Geometry check sheet. Reference: the model listing, model coordinates, mm. A direction names the side the tool comes from. Coordinates: 2 decimals unless noted, no trailing zeros. Write each loop counter-clockwise with the first axis right and the second up, starting at its lowest first coordinate (ties: lowest second). Pieces come first, ordered by that corner, then holes. Notation, with made-up numbers: M -7,-18.75 L 19,-18.75 A16 cw 19,8.25 Z; hole C 46.25,-35.75 d7. An arc over 180 degrees is marked long. Put each result on its own line as item: value. Start each with the question number.
1) Set-up check for faces 5 (the flat face through (-31.5, 1.4, 25.7)), 6 (the flat face through (-9.563, 1.401, 22.927)), 7 (the flat face through (-9.563, -1.401, 22.927)): record each of +Z, -Z, +X, -X, +Y, -Y from which the full face is reachable in a straight line by a thin tool's end or side.
2) Scan lines: line 1 along Y through (x, z) = (-2.5, -5.5); line 2 along Y through (x, z) = (-16, 17). Record each from-to range of solid material in increasing order.
3) Gauge pin test, flat ends, axial feed: pin 1 (1 mm diameter, centred on x = -0.5, z = 5.5, fed in from -Y); pin 2 (12 mm diameter, centred on x = -1, z = -2, fed in from -Y); pin 3 (1.5 mm diameter, centred on x = -41.5, y = -1.5, fed in from -Z). Record the tip position at first contact, or that the pin passes through.
4) Mould release check, pull along X, two halves, no side actions. Record for faces 1 (the flat face through (-9.52, -1.98, -1.27)), 2 (the flat face through (-4.314, -1.586, 21.033)), 3 (the flat face through (-10.107, 1.586, 21.141)), 4 (the flat face through (17.372, -1.586, 24.768)): released by +X, released by -X, zero draft, split by the parting line, or undercut.
5) Cross-section at B-B on z = -1. Record the cut outline in (x, y), plus the area to 3 significant figures.
6) Cross-section at A-A on z = 25.5. Count the separate pieces of the cut face and the enclosed holes in it, plus the area to 3 significant figures.
from build123d import *


with BuildPart() as f3:
    # F0 (on Front) → F3 section 0
    with BuildSketch(Plane.XZ, mode=Mode.PRIVATE) as f3_s0:
        with BuildLine():
            Line((-21.9142735004, 32.6593369246), (-64.6117627621, 32.6593369246))
            add(Edge.make_bspline(
                [(-64.6117627621, 32.6593369246), (-63.1112154786, 31.6044133494), (-59.4897111338, 29.4798106269), (-54.8402694545, 24.0083886157), (-54.1776311477, 17.803548493), (-53.0184023082, 15.6934484839)],
                knots=[0, 0, 0, 0, 0.3044179075, 0.6380886555, 1, 1, 1, 1], degree=3))
            add(Edge.make_bspline(
                [(-53.0184023082, 15.6934484839), (-50.397152359, 15.9517944961), (-42.4564652069, 16.5735141568), (-30.3318480055, 11.9726995365), (-22.6326325716, 7.7807102957), (-19.3285813991, 1.5879180834), (-17.1072725207, 0)],
                knots=[0, 0, 0, 0, 0.2494885994, 0.5320392712, 0.7637954486, 1, 1, 1, 1], degree=3))
            Line((-17.1072725207, 0), (-7.2105028667, -11.7347398773))
            Line((-7.2105028667, -11.7347398773), (2.6862667874, 0))
            add(Edge.make_bspline(
                [(38.5973965749, 15.6934484839), (35.9761466257, 15.9517944961), (28.0354594736, 16.5735141568), (15.9108422722, 11.9726995365), (8.2116268383, 7.7807102957), (4.9075756658, 1.5879180834), (2.6862667874, 0)],
                knots=[0, 0, 0, 0, 0.2494885994, 0.5320392712, 0.7637954486, 1, 1, 1, 1], degree=3))
            add(Edge.make_bspline(
                [(50.1907570288, 32.6593369246), (48.6902097453, 31.6044133494), (45.0687054005, 29.4798106269), (40.4192637212, 24.0083886157), (39.7566254144, 17.803548493), (38.5973965749, 15.6934484839)],
                knots=[0, 0, 0, 0, 0.3044179075, 0.6380886555, 1, 1, 1, 1], degree=3))
            Line((50.1907570288, 32.6593369246), (7.4932677671, 32.6593369246))
            add(Edge.make_bspline(
                [(7.4932677671, 32.6593369246), (7.7789275206, 30.681626577), (8.3182882425, 26.9541985329), (4.3276740221, 24.1005648406), (-0.3013873529, 24.1408897918), (-2.9690302908, 24.1763927042)],
                knots=[0, 0, 0, 0, 0.3305961482, 0.6143190537, 1, 1, 1, 1], degree=3))
            Line((-2.9690302908, 24.1763927042), (-2.9690302908, 30.962748453))
            Line((-2.9690302908, 30.962748453), (-4.662130028, 27.2415857762))
            Line((-4.662130028, 27.2415857762), (-7.2105028667, 27.2415857762))
            Line((-7.2105028667, 27.2415857762), (-9.7588757053, 27.2415857762))
            Line((-9.7588757053, 27.2415857762), (-11.4519754425, 30.962748453))
            Line((-11.4519754425, 30.962748453), (-11.4519754425, 24.1763927042))
            add(Edge.make_bspline(
                [(-21.9142735004, 32.6593369246), (-22.199933254, 30.681626577), (-22.7392939758, 26.9541985329), (-18.7486797554, 24.1005648406), (-14.1196183804, 24.1408897918), (-11.4519754425, 24.1763927042)],
                knots=[0, 0, 0, 0, 0.3305961482, 0.6143190537, 1, 1, 1, 1], degree=3))
        make_face()
    loft([f3_s0.sketch, Vertex(-7.2105028667, -5, 7.7760326676)])

    # F0 (on Front) → F6 section 0
    with BuildSketch(Plane.XZ, mode=Mode.PRIVATE) as f6_s0:
        with BuildLine():
            Line((-21.9142735004, 32.6593369246), (-64.6117627621, 32.6593369246))
            add(Edge.make_bspline(
                [(-64.6117627621, 32.6593369246), (-63.1112154786, 31.6044133494), (-59.4897111338, 29.4798106269), (-54.8402694545, 24.0083886157), (-54.1776311477, 17.803548493), (-53.0184023082, 15.6934484839)],
                knots=[0, 0, 0, 0, 0.3044179075, 0.6380886555, 1, 1, 1, 1], degree=3))
            add(Edge.make_bspline(
                [(-53.0184023082, 15.6934484839), (-50.397152359, 15.9517944961), (-42.4564652069, 16.5735141568), (-30.3318480055, 11.9726995365), (-22.6326325716, 7.7807102957), (-19.3285813991, 1.5879180834), (-17.1072725207, 0)],
                knots=[0, 0, 0, 0, 0.2494885994, 0.5320392712, 0.7637954486, 1, 1, 1, 1], degree=3))
            Line((-17.1072725207, 0), (-7.2105028667, -11.7347398773))
            Line((-7.2105028667, -11.7347398773), (2.6862667874, 0))
            add(Edge.make_bspline(
                [(38.5973965749, 15.6934484839), (35.9761466257, 15.9517944961), (28.0354594736, 16.5735141568), (15.9108422722, 11.9726995365), (8.2116268383, 7.7807102957), (4.9075756658, 1.5879180834), (2.6862667874, 0)],
                knots=[0, 0, 0, 0, 0.2494885994, 0.5320392712, 0.7637954486, 1, 1, 1, 1], degree=3))
            add(Edge.make_bspline(
                [(50.1907570288, 32.6593369246), (48.6902097453, 31.6044133494), (45.0687054005, 29.4798106269), (40.4192637212, 24.0083886157), (39.7566254144, 17.803548493), (38.5973965749, 15.6934484839)],
                knots=[0, 0, 0, 0, 0.3044179075, 0.6380886555, 1, 1, 1, 1], degree=3))
            Line((50.1907570288, 32.6593369246), (7.4932677671, 32.6593369246))
            add(Edge.make_bspline(
                [(7.4932677671, 32.6593369246), (7.7789275206, 30.681626577), (8.3182882425, 26.9541985329), (4.3276740221, 24.1005648406), (-0.3013873529, 24.1408897918), (-2.9690302908, 24.1763927042)],
                knots=[0, 0, 0, 0, 0.3305961482, 0.6143190537, 1, 1, 1, 1], degree=3))
            Line((-2.9690302908, 24.1763927042), (-2.9690302908, 30.962748453))
            Line((-2.9690302908, 30.962748453), (-4.662130028, 27.2415857762))
            Line((-4.662130028, 27.2415857762), (-7.2105028667, 27.2415857762))
            Line((-7.2105028667, 27.2415857762), (-9.7588757053, 27.2415857762))
            Line((-9.7588757053, 27.2415857762), (-11.4519754425, 30.962748453))
            Line((-11.4519754425, 30.962748453), (-11.4519754425, 24.1763927042))
            add(Edge.make_bspline(
                [(-21.9142735004, 32.6593369246), (-22.199933254, 30.681626577), (-22.7392939758, 26.9541985329), (-18.7486797554, 24.1005648406), (-14.1196183804, 24.1408897918), (-11.4519754425, 24.1763927042)],
                knots=[0, 0, 0, 0, 0.3305961482, 0.6143190537, 1, 1, 1, 1], degree=3))
        make_face()
    loft([f6_s0.sketch, Vertex(-7.2105028667, 5, 7.7760326676)])


solid = f3.part
Answer key:
1. face 5: +Z, +X, -X, +Y
1. face 6: +Z, +Y
1. face 7: +Z, -Y
2. line 1: y = -0.17 to 0.17
2. line 2: y = -3.15 to 3.15
3. pin 1: stops at y = -2.62
3. pin 2: stops at y = -2.99
3. pin 3: stops at z = 13.58
4. face 1: released by -X
4. face 2: undercut
4. face 3: undercut
4. face 4: zero draft
5. outline: M -16.26,0 L -7.21,-2.75 L 1.84,0 L -7.21,2.75 Z
5. area: 49.8 mm²
6. separate pieces: 3
6. enclosed holes: 0
6. area: 194 mm²
